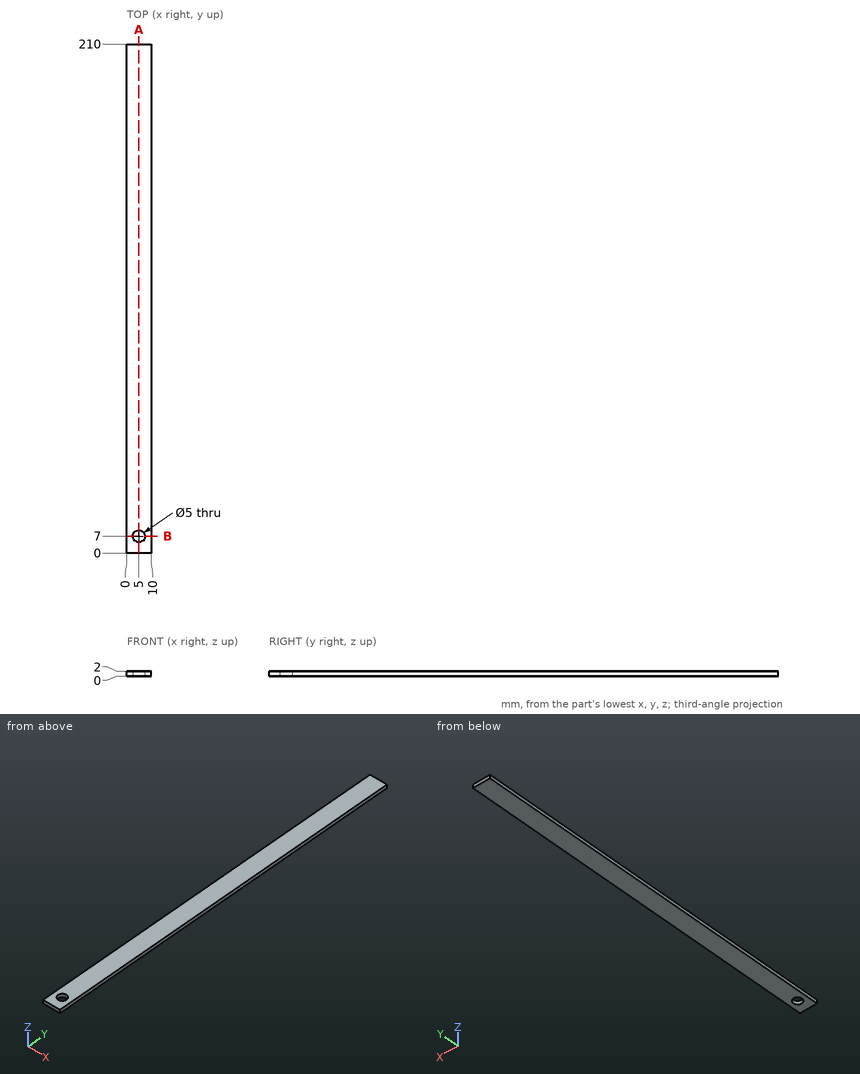
Could you check a few things on this drawing? It's one solid part, dimensions in mm from its lowest x, y, z. Give positions to 0.01 mm unless a question says otherwise; leave off trailing zeros. Loops run counter-clockwise (first coordinate to the right, second up) from the corner with the lowest first, then second, coordinate; pieces in that order, holes last. Notation, with made-up numbers: M 61,18 L 96,18 A16 cw 96,37 Z; hole C -25.75,7.25 d2. An arc over 180 degrees is marked long. One line per question, with ' | ' between items. Start each with the question number.
Q1. If I drill on line 1 (X direction, y = 7, z = 1.55); line 2 (Y direction, x = 5, z = 1.65); line 3 (Y direction, x = 6, z = 1.55), over which ranges is the centre line in solid material (lowest first)? Write a range as from..to.
Q2. For pin 1 Ø1 at (x, y) = (5.5, 132.5) entering from -Z, with a flat end and sliding along its axis, tell me the tip position at first contact or that it passes through.
Q3. If we section it at B-B (y = 7): Please give me the cut outline in (x, z), plus the area to 3 significant figures.
Q4. If we section it at A-A (x = 5): Please give me the cut outline in (y, z).
Computed:
1) line 1: x = 0..2.5, 7.5..10 | line 2: y = 0..4.5, 9.5..210 | line 3: y = 0..4.71, 9.29..210
2) pin 1: stops at z = 0
3) outline: M 0,0 L 2.5,0 L 2.5,2 L 0,2 Z; M 7.5,0 L 10,0 L 10,2 L 7.5,2 Z | area: 10.0 mm²
4) outline: M 0,0 L 4.5,0 L 4.5,2 L 0,2 Z; M 9.5,0 L 210,0 L 210,2 L 9.5,2 Z
